Input: part model. Units: mm. Frame: model coordinates. A direction names the side the tool comes from. Round coordinates to 2 decimals unless told otherwise and drop trailing zeros. Order: outer loops, then holes, each group sorted by start corner. A loop starts at its lowest first (then second) coordinate and runs counter-clockwise, first axis right, second up. Notation, with made-up numbers: (-10.75, 57) -> (-3.75, 57) arc R18 ccw to (-3.75, 62) -> close; hole circle Ø3 at (49.5, 30.5). An arc over 180 degrees is marked (long way). Use a Markdown table: item, result.
from build123d import *

# Parameters (mm, degrees)
F1_DEPTH = 25
F3_D     = 3.3
F4_W     = 10
F4_H     = 30
F5_DEPTH = 2
F6_D     = 4.4
F7_DEPTH = 2
F8_R     = 3


with BuildPart() as f1:
    # F0 (on Right) → F1 (new body, symmetric)
    with BuildSketch(Plane.YZ):
        with BuildLine():
            ThreePointArc((-5, 0), (-1.4644660941, 1.4644660941), (0, 5))
            Line((0, 5), (0, 40))
            Line((0, 40), (-2, 40))
            Line((-2, 40), (-2, 5))
            ThreePointArc((-2, 5), (-2.8786796564, 2.8786796564), (-5, 2))
            Line((-5, 2), (-52, 2))
            Line((-52, 2), (-52, 0))
            Line((-52, 0), (-5, 0))
        make_face()
    extrude(amount=F1_DEPTH, both=True)

    # F3 (through all)
    with Locations(Plane.XZ.offset(2)):
        with Locations((-15, 32.5), (-15, 11), (15, 11), (15, 32.5)):
            Hole(F3_D / 2)

    # F4 (on face) → F5 (join, through all)
    with BuildSketch(Plane.XY.offset(2)):
        with Locations((-30, -37)):
            Rectangle(F4_W, F4_H)
        with Locations((30, -37)):
            Rectangle(F4_W, F4_H)
    extrude(amount=-F5_DEPTH)

    # F6 (through all)
    with Locations(Plane.XY.offset(2)):
        with Locations((-25, -38), (25, -38)):
            Hole(F6_D / 2)

    # F4 (on face) → F7 (cut, through all)
    with BuildSketch(Plane.XY.offset(2)):
        with BuildLine():
            ThreePointArc((15, -37), (0, -22), (-15, -37))
            ThreePointArc((-15, -37), (-10.6066017178, -47.6066017178), (0, -52))
            ThreePointArc((0, -52), (10.6066017178, -47.6066017178), (15, -37))
        make_face()
        with BuildLine():
            Line((-15, -37), (-15, -52))
            Line((-15, -52), (0, -52))
            ThreePointArc((0, -52), (-10.6066017178, -47.6066017178), (-15, -37))
        make_face()
        with BuildLine():
            ThreePointArc((15, -37), (10.6066017178, -47.6066017178), (0, -52))
            Line((0, -52), (15, -52))
            Line((15, -52), (15, -37))
        make_face()
    extrude(amount=-F7_DEPTH, mode=Mode.SUBTRACT)

    # F8
    f8_edges = [f1.edges().sort_by_distance(p)[0] for p in [
        (-15, -52, 1),
        (-35, -52, 1),
        (-35, -22, 1),
        (-25, -22, 1),
        (-25, -1, 40),
        (15, -52, 1),
        (35, -52, 1),
        (35, -22, 1),
        (25, -22, 1),
        (25, -1, 40),
    ]]
    fillet(f8_edges, radius=F8_R)


solid = f1.part
1) Contact query for flat-ended pins moving along their axis: P1, Ø2.5, axis at x = 15, z = 32.5, coming from the -Y side; P2, Ø7, axis at x = 25, y = -38, coming from the +Z side; P3, Ø0.6, axis at x = -30, z = 0.5, coming from the +Y side; P4, Ø17.5, axis at x = 9, z = 22.5, coming from the -Y side. Output: stop coordinate, or through.
Answer key:
| item | result |
|---|---|
| P1 | passes through |
| P2 | stops at z = 2 |
| P3 | stops at y = -22 |
| P4 | stops at y = -2 |
2) Cut plane D-D on y = -15.5. Return loops of the section in (x, z).
Answer key:
| item | result |
|---|---|
| outline | (-25, 0) -> (25, 0) -> (25, 2) -> (-25, 2) -> close |
3) Set-up query: faces 1 (the face through (7, -23, 2)), 2 (the face through (25, -1.8, 15.8)), 3 (the face through (15, -43, 1)), 4 (the face through (-30, -22, 1)). Return all of +Z, -Z, +X, -X, +Y, -Y with unobstructed straight access to the full face (end or side cutting, diameter ignored); none if empty.
Answer key:
| item | result |
|---|---|
| face 1 | +Z, +X, -X, -Y |
| face 2 | +Z, -Z, +X, +Y |
| face 3 | +Z, -Z, -Y |
| face 4 | +Z, -Z, -X, +Y |
4) Draft query along X for faces 5 (the face through (25.86, -21.1, 0.99)), 6 (the face through (-25.9, -21.14, 0.99)), 7 (the face through (-15.89, -0.99, 33.89)), 8 (the face through (25.477, -40.148, 0.986)). Return one class per face: released by +X, released by -X, zero draft, split by the parting line, or undercut.
Answer key:
| item | result |
|---|---|
| face 5 | released by +X |
| face 6 | released by -X |
| face 7 | undercut |
| face 8 | undercut |
5) Cut plane A-A on y = -38. Return loops of the section in (x, z), and give its area (3 significant figures).
Answer key:
| item | result |
|---|---|
| outline | (-35, 0) -> (-27.2, 0) -> (-27.2, 2) -> (-35, 2) -> close; (-22.8, 0) -> (-15, 0) -> (-15, 2) -> (-22.8, 2) -> close; (15, 0) -> (22.8, 0) -> (22.8, 2) -> (15, 2) -> close; (27.2, 0) -> (35, 0) -> (35, 2) -> (27.2, 2) -> close |
| area | 62.4 mm^2 |
6) Cut plane B-B on z = 32.5. Return loops of the section in (x, y), and give its area (3 significant figures).
Answer key:
| item | result |
|---|---|
| outline | (-25, -2) -> (-16.65, -2) -> (-16.65, 0) -> (-25, 0) -> close; (-13.35, -2) -> (13.35, -2) -> (13.35, 0) -> (-13.35, 0) -> close; (16.65, -2) -> (25, -2) -> (25, 0) -> (16.65, 0) -> close |
| area | 86.8 mm^2 |
7) Cut plane C-C on x = -20. Return loops of the section in (y, z).
Answer key:
| item | result |
|---|---|
| outline | (-52, 0) -> (-5, 0) arc R5 ccw to (0, 5) -> (0, 40) -> (-2, 40) -> (-2, 5) arc R3 cw to (-5, 2) -> (-52, 2) -> close |
8) Ray query, probe 1 along Z at (x, y) = (6.5, -16.5); probe 2 along Y at (x, z) = (15, 25.5); probe 3 along Z at (x, y) = (15, -1.45). Return the intervals inside material, ascending.
Answer key:
| item | result |
|---|---|
| probe 1 | z = 0 to 2 |
| probe 2 | y = -2 to 0 |
| probe 3 | z = 1.48 to 9.35, 12.65 to 30.85, 34.15 to 40 |
